Drawing for the job (mm, zero at the part's lowest x, y, z). A direction names the side the tool comes from. Round coordinates to 2 decimals unless told otherwise and drop trailing zeros. Write each loop counter-clockwise with the first axis right and the second up, starting at its lowest first coordinate (ties: lowest second). Pieces come first, ordered by that corner, then holes. Notation, with made-up numbers: (65.25, 29.5) - (105.25, 29.5) arc R31 ccw to (105.25, 65.5) - close; hole circle Ø7 at (-35.75, 12). An arc over 180 degrees is marked (long way). Answer in a Markdown table with one row per item.
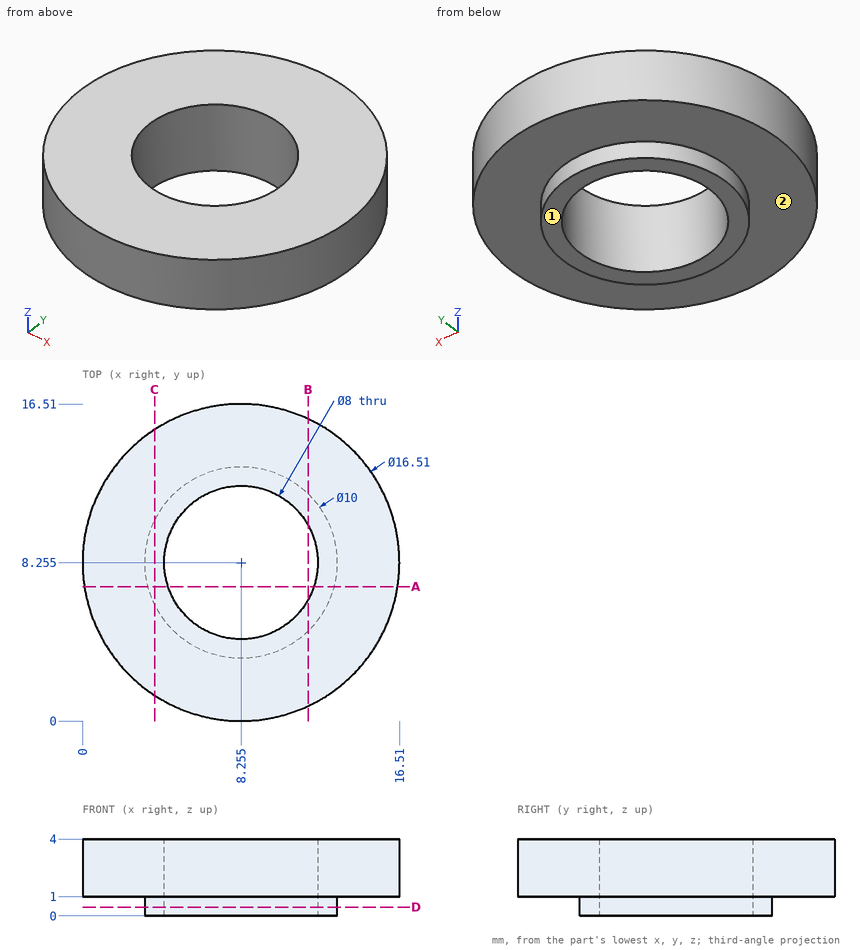
Q1. Saw through at A-A on y = 7. List the corners of the cut face in (x, z).
Computed:
| item | result |
|---|---|
| outline | (0.1, 1) - (3.42, 1) - (3.42, 0) - (4.46, 0) - (4.46, 4) - (0.1, 4) - close; (12.05, 0) - (13.09, 0) - (13.09, 1) - (16.41, 1) - (16.41, 4) - (12.05, 4) - close |
Q2. Saw through at C-C on x = 3.75. List the corners of the cut face in (y, z).
Computed:
| item | result |
|---|---|
| outline | (1.34, 1) - (6.09, 1) - (6.09, 0) - (10.42, 0) - (10.42, 1) - (15.17, 1) - (15.17, 4) - (1.34, 4) - close |
Q3. 3-axis set-ups, long thin cutter, end or side, ignore diameter. For the marked faces 1 and 2: which of +Z, -Z, +X, -X, +Y, -Y reach the whole face in a straight line?
Computed:
| item | result |
|---|---|
| face 1 | -Z, +X, -X, +Y, -Y |
| face 2 | -Z |
Q4. Drill centre lines: line 1 (Z direction, x = 2.25, y = 10); line 2 (X direction, y = 8.75, z = 0.8); line 3 (X direction, y = 10.5, z = 0.35). Where is each one in solid material? Low to high.
Computed:
| item | result |
|---|---|
| line 1 | z = 1 to 4 |
| line 2 | x = 3.28 to 4.29, 12.22 to 13.23 |
| line 3 | x = 3.79 to 4.94, 11.57 to 12.72 |
Q5. Saw through at B-B on x = 11.75. List the corners of the cut face in (y, z).
Computed:
| item | result |
|---|---|
| outline | (0.78, 1) - (4.68, 1) - (4.68, 0) - (6.31, 0) - (6.31, 4) - (0.78, 4) - close; (10.2, 0) - (11.83, 0) - (11.83, 1) - (15.73, 1) - (15.73, 4) - (10.2, 4) - close |
Q6. Saw through at D-D on z = 0.45. List the corners of the cut face in (x, y) (3 decimals).
Computed:
| item | result |
|---|---|
| outline | circle Ø10 at (8.255, 8.255); hole circle Ø8 at (8.255, 8.255) |
Q7. Flat gauge pins, fed straight in: pin 1 (1 mm diameter, centred on y = 14.5, z = 1, fed in from -X); pin 2 (3 mm diameter, centred on x = 8.5, y = 13.5, fed in from -Z); pin 3 (1.5 mm diameter, centred on x = 4.5, z = 3.5, fed in from -Y). Where does each tip first touch, or does it go through?
Computed:
| item | result |
|---|---|
| pin 1 | stops at x = 2.33 |
| pin 2 | stops at z = 0 |
| pin 3 | stops at y = 0.57 |
